Source: CAD feature listing. Evaluate the final solid. Frame: model axes, mm. Face numbers are marked on the shaded views. Give positions to 0.01 mm unless a question says otherwise; leave off trailing zeros. Loops run counter-clockwise (first coordinate to the right, second up) from the corner with the lowest first, then second, coordinate; pieces in that order, holes last. Notation, with made-up numbers: M 85,63 L 134,63 A22 cw 134,84 Z; hole C 63.5,10 d8. An arc over 180 degrees is marked long. Put each result on its own line as item: value. Start each with the question number.
```python
from build123d import *

# Parameters (mm, degrees)
F1_DEPTH = 5
F2_DEPTH = 15
F3_DEPTH = 22


with BuildPart() as f1:
    # F0 (on Top) → F1 (new body)
    with BuildSketch(Plane.XY):
        with BuildLine():
            ThreePointArc((-49.4411764706, 56.0621778265), (-46.8789986441, 53.5), (-45.9411764706, 50))
            ThreePointArc((-45.9411764706, 50), (-46.8789986441, 46.5), (-49.4411764706, 43.9378221735))
            ThreePointArc((-49.4411764706, 43.9378221735), (-52.9411764706, 43), (-56.4411764706, 43.9378221735))
            ThreePointArc((-56.4411764706, 43.9378221735), (-59.0033542971, 46.5), (-59.9411764706, 50))
            Line((-59.9411764706, 50), (-59.9411764706, -50))
            ThreePointArc((-59.9411764706, -50), (-59.0033542971, -46.5), (-56.4411764706, -43.9378221735))
            ThreePointArc((-56.4411764706, -43.9378221735), (-52.9411764706, -43), (-49.4411764706, -43.9378221735))
            ThreePointArc((-49.4411764706, -43.9378221735), (-46.8789986441, -46.5), (-45.9411764706, -50))
            ThreePointArc((-45.9411764706, -50), (-46.8789986441, -53.5), (-49.4411764706, -56.0621778265))
            ThreePointArc((-49.4411764706, -56.0621778265), (-51.1294431549, -56.761480784), (-52.9411764706, -57))
            Line((-52.9411764706, -57), (47.0588235294, -57))
            ThreePointArc((47.0588235294, -57), (45.2470902137, -56.761480784), (43.5588235294, -56.0621778265))
            ThreePointArc((43.5588235294, -56.0621778265), (40.9966457029, -53.5), (40.0588235294, -50))
            ThreePointArc((40.0588235294, -50), (40.9966457029, -46.5), (43.5588235294, -43.9378221735))
            ThreePointArc((43.5588235294, -43.9378221735), (47.0588235294, -43), (50.5588235294, -43.9378221735))
            ThreePointArc((50.5588235294, -43.9378221735), (53.1210013559, -46.5), (54.0588235294, -50))
            Line((54.0588235294, -50), (54.0588235294, 50))
            ThreePointArc((54.0588235294, 50), (53.1210013559, 46.5), (50.5588235294, 43.9378221735))
            ThreePointArc((50.5588235294, 43.9378221735), (47.0588235294, 43), (43.5588235294, 43.9378221735))
            ThreePointArc((43.5588235294, 43.9378221735), (40.9966457029, 46.5), (40.0588235294, 50))
            ThreePointArc((40.0588235294, 50), (40.9966457029, 53.5), (43.5588235294, 56.0621778265))
            ThreePointArc((43.5588235294, 56.0621778265), (45.2470902137, 56.761480784), (47.0588235294, 57))
            Line((47.0588235294, 57), (-52.9411764706, 57))
            ThreePointArc((-52.9411764706, 57), (-51.1294431549, 56.761480784), (-49.4411764706, 56.0621778265))
        make_face()
    extrude(amount=F1_DEPTH)

    # F0 (on Top) → F2 (join)
    with BuildSketch(Plane.XY):
        Polygon((-49.4411764706, 43.9378221735), (-45.9411764706, 50), (-49.4411764706, 56.0621778265), (-56.4411764706, 56.0621778265), (-59.9411764706, 50), (-56.4411764706, 43.9378221735), align=None)
        Polygon((50.5588235294, -56.0621778265), (54.0588235294, -50), (50.5588235294, -43.9378221735), (43.5588235294, -43.9378221735), (40.0588235294, -50), (43.5588235294, -56.0621778265), align=None)
        Polygon((-56.4411764706, -43.9378221735), (-59.9411764706, -50), (-56.4411764706, -56.0621778265), (-49.4411764706, -56.0621778265), (-45.9411764706, -50), (-49.4411764706, -43.9378221735), align=None)
        with BuildLine():
            ThreePointArc((50.5588235294, -56.0621778265), (53.1210013559, -53.5), (54.0588235294, -50))
            Line((54.0588235294, -50), (50.5588235294, -56.0621778265))
        make_face()
        with BuildLine():
            Line((43.5588235294, -43.9378221735), (50.5588235294, -43.9378221735))
            ThreePointArc((50.5588235294, -43.9378221735), (47.0588235294, -43), (43.5588235294, -43.9378221735))
        make_face()
        with BuildLine():
            Line((40.0588235294, -50), (43.5588235294, -43.9378221735))
            ThreePointArc((43.5588235294, -43.9378221735), (40.9966457029, -46.5), (40.0588235294, -50))
        make_face()
        with BuildLine():
            ThreePointArc((40.0588235294, -50), (40.9966457029, -53.5), (43.5588235294, -56.0621778265))
            Line((43.5588235294, -56.0621778265), (40.0588235294, -50))
        make_face()
        with BuildLine():
            ThreePointArc((-45.9411764706, -50), (-46.8789986441, -46.5), (-49.4411764706, -43.9378221735))
            Line((-49.4411764706, -43.9378221735), (-45.9411764706, -50))
        make_face()
        with BuildLine():
            ThreePointArc((-49.4411764706, -43.9378221735), (-52.9411764706, -43), (-56.4411764706, -43.9378221735))
            Line((-56.4411764706, -43.9378221735), (-49.4411764706, -43.9378221735))
        make_face()
        with BuildLine():
            Line((-45.9411764706, -50), (-49.4411764706, -56.0621778265))
            ThreePointArc((-49.4411764706, -56.0621778265), (-46.8789986441, -53.5), (-45.9411764706, -50))
        make_face()
        with BuildLine():
            ThreePointArc((-56.4411764706, -43.9378221735), (-59.0033542971, -46.5), (-59.9411764706, -50))
            Line((-59.9411764706, -50), (-56.4411764706, -43.9378221735))
        make_face()
        with BuildLine():
            Line((-49.4411764706, -56.0621778265), (-56.4411764706, -56.0621778265))
            ThreePointArc((-56.4411764706, -56.0621778265), (-54.7529097863, -56.761480784), (-52.9411764706, -57))
            ThreePointArc((-52.9411764706, -57), (-51.1294431549, -56.761480784), (-49.4411764706, -56.0621778265))
        make_face()
        with BuildLine():
            Line((-56.4411764706, -56.0621778265), (-59.9411764706, -50))
            ThreePointArc((-59.9411764706, -50), (-59.0033542971, -53.5), (-56.4411764706, -56.0621778265))
        make_face()
        with BuildLine():
            Line((-56.4411764706, 56.0621778265), (-49.4411764706, 56.0621778265))
            ThreePointArc((-49.4411764706, 56.0621778265), (-51.1294431549, 56.761480784), (-52.9411764706, 57))
            ThreePointArc((-52.9411764706, 57), (-54.7529097863, 56.761480784), (-56.4411764706, 56.0621778265))
        make_face()
        with BuildLine():
            Line((-49.4411764706, 56.0621778265), (-45.9411764706, 50))
            ThreePointArc((-45.9411764706, 50), (-46.8789986441, 53.5), (-49.4411764706, 56.0621778265))
        make_face()
        with BuildLine():
            ThreePointArc((-49.4411764706, 43.9378221735), (-46.8789986441, 46.5), (-45.9411764706, 50))
            Line((-45.9411764706, 50), (-49.4411764706, 43.9378221735))
        make_face()
        with BuildLine():
            Line((-59.9411764706, 50), (-56.4411764706, 56.0621778265))
            ThreePointArc((-56.4411764706, 56.0621778265), (-59.0033542971, 53.5), (-59.9411764706, 50))
        make_face()
        with BuildLine():
            ThreePointArc((-59.9411764706, 50), (-59.0033542971, 46.5), (-56.4411764706, 43.9378221735))
            Line((-56.4411764706, 43.9378221735), (-59.9411764706, 50))
        make_face()
        with BuildLine():
            ThreePointArc((-56.4411764706, 43.9378221735), (-52.9411764706, 43), (-49.4411764706, 43.9378221735))
            Line((-49.4411764706, 43.9378221735), (-56.4411764706, 43.9378221735))
        make_face()
        with BuildLine():
            ThreePointArc((50.5588235294, 56.0621778265), (48.8705568451, 56.761480784), (47.0588235294, 57))
            ThreePointArc((47.0588235294, 57), (45.2470902137, 56.761480784), (43.5588235294, 56.0621778265))
            Line((43.5588235294, 56.0621778265), (50.5588235294, 56.0621778265))
        make_face()
        with BuildLine():
            ThreePointArc((54.0588235294, 50), (53.1210013559, 53.5), (50.5588235294, 56.0621778265))
            Line((50.5588235294, 56.0621778265), (54.0588235294, 50))
        make_face()
        with BuildLine():
            ThreePointArc((50.5588235294, 43.9378221735), (53.1210013559, 46.5), (54.0588235294, 50))
            Line((54.0588235294, 50), (50.5588235294, 43.9378221735))
        make_face()
        with BuildLine():
            ThreePointArc((43.5588235294, 43.9378221735), (47.0588235294, 43), (50.5588235294, 43.9378221735))
            Line((50.5588235294, 43.9378221735), (43.5588235294, 43.9378221735))
        make_face()
        with BuildLine():
            Line((43.5588235294, 43.9378221735), (40.0588235294, 50))
            ThreePointArc((40.0588235294, 50), (40.9966457029, 46.5), (43.5588235294, 43.9378221735))
        make_face()
        with BuildLine():
            Line((40.0588235294, 50), (43.5588235294, 56.0621778265))
            ThreePointArc((43.5588235294, 56.0621778265), (40.9966457029, 53.5), (40.0588235294, 50))
        make_face()
        Polygon((54.0588235294, 50), (50.5588235294, 56.0621778265), (43.5588235294, 56.0621778265), (40.0588235294, 50), (43.5588235294, 43.9378221735), (50.5588235294, 43.9378221735), align=None)
        with BuildLine():
            ThreePointArc((47.0588235294, -57), (48.8705568451, -56.761480784), (50.5588235294, -56.0621778265))
            Line((50.5588235294, -56.0621778265), (43.5588235294, -56.0621778265))
            ThreePointArc((43.5588235294, -56.0621778265), (45.2470902137, -56.761480784), (47.0588235294, -57))
        make_face()
        with BuildLine():
            Line((50.5588235294, -43.9378221735), (54.0588235294, -50))
            ThreePointArc((54.0588235294, -50), (53.1210013559, -46.5), (50.5588235294, -43.9378221735))
        make_face()
    extrude(amount=F2_DEPTH)

    # F0 (on Top) → F3 (join)
    with BuildSketch(Plane.XY):
        Polygon((-49.4411764706, 43.9378221735), (-45.9411764706, 50), (-49.4411764706, 56.0621778265), (-56.4411764706, 56.0621778265), (-59.9411764706, 50), (-56.4411764706, 43.9378221735), align=None)
        Polygon((50.5588235294, -56.0621778265), (54.0588235294, -50), (50.5588235294, -43.9378221735), (43.5588235294, -43.9378221735), (40.0588235294, -50), (43.5588235294, -56.0621778265), align=None)
        Polygon((-56.4411764706, -43.9378221735), (-59.9411764706, -50), (-56.4411764706, -56.0621778265), (-49.4411764706, -56.0621778265), (-45.9411764706, -50), (-49.4411764706, -43.9378221735), align=None)
        Polygon((54.0588235294, 50), (50.5588235294, 56.0621778265), (43.5588235294, 56.0621778265), (40.0588235294, 50), (43.5588235294, 43.9378221735), (50.5588235294, 43.9378221735), align=None)
    extrude(amount=F3_DEPTH)


solid = f1.part
```
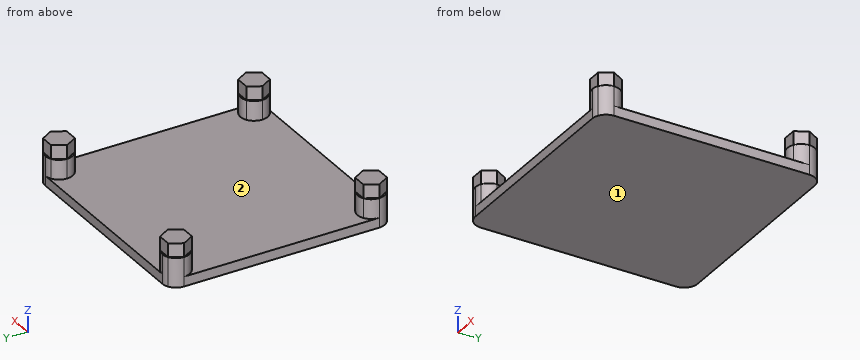
1. Section A-A, the plane z = 7.75. Output: boundary loops of the cut face in (x, y), plus the area to 3 significant figures.
2. Section B-B, the plane y = 48. Output: boundary loops of the cut face in (x, z).
3. Section C-C, the plane z = 17.5. Output: boundary loops of the cut face in (x, y), plus the area to 3 significant figures.
4. Pull-direction query (Y, two-part tool) for the marked faces 1 and 2; classes: released by +Y, released by -Y, zero draft, split by the parting line, or undercut.
5. Ray query, line 1 (Z direction, x = -9.5, y = 0); line 2 (Y direction, x = -46.5, z = 15.25); line 3 (X direction, y = -44.5, z = 18.75). Return the intervals inside material, ascending.
6. Section D-D, the plane x = -33.5. Output: boundary loops of the cut face in (y, z).
7. Contact query for flat-ended pins moving along their axis: pin 1 (3.5 mm diameter, centred on x = 45.5, z = 19.5, fed in from -Y); pin 2 (3 mm diameter, centred on x = -7, y = 19.5, fed in from +Z); pin 3 (2 mm diameter, centred on x = -52.5, z = 17.5, fed in from +Y). Output: stop coordinate, or through.
Results found:
1. outline: C -52.94,-50 d14; C -52.94,50 d14; C 47.06,-50 d14; C 47.06,50 d14
1. area: 616 mm²
2. outline: M -59.94,0 L 54.06,0 L 54.06,5 L 53.77,5 L 53.77,15 L 52.9,15 L 52.9,22 L 41.21,22 L 41.21,15 L 40.35,15 L 40.35,5 L -46.23,5 L -46.23,15 L -47.1,15 L -47.1,22 L -58.79,22 L -58.79,15 L -59.65,15 L -59.65,5 L -59.94,5 Z
3. outline: M -59.94,-50 L -56.44,-56.06 L -49.44,-56.06 L -45.94,-50 L -49.44,-43.94 L -56.44,-43.94 Z; M -59.94,50 L -56.44,43.94 L -49.44,43.94 L -45.94,50 L -49.44,56.06 L -56.44,56.06 Z; M 40.06,-50 L 43.56,-56.06 L 50.56,-56.06 L 54.06,-50 L 50.56,-43.94 L 43.56,-43.94 Z; M 40.06,50 L 43.56,43.94 L 50.56,43.94 L 54.06,50 L 50.56,56.06 L 43.56,56.06 Z
3. area: 509 mm²
4. face 1: zero draft
4. face 2: undercut
5. line 1: 0 to 5
5. line 2: -50.97 to -49.03, 49.03 to 50.97
5. line 3: -56.77 to -49.12, 43.23 to 50.88
6. outline: M -57,0 L 57,0 L 57,5 L -57,5 Z
7. pin 1: y = -56.06
7. pin 2: z = 5
7. pin 3: y = 56.06
